For this review, take the finished solid that the model builds, in its own axes (mm). Face numbers are marked on the shaded views. A direction names the side the tool comes from. Give positions to 0.01 mm unless a question says otherwise; leave off trailing zeros. Loops run counter-clockwise (first coordinate to the right, second up) from the corner with the lowest first, then second, coordinate; pieces in that order, holes last. Notation, with made-up numbers: (-35.5, 66.25) -> (13.5, 66.25) arc R23 ccw to (13.5, 101.25) -> close; hole circle Ø11 at (12, 40.5). An arc over 180 degrees is marked (long way). Answer as CSV lines item,"result". Start each with the question number.
Item 1: For L1, parallel to Z at x = 0, y = -6; L2, parallel to Z at x = 1.75, y = 4; L3, parallel to X at y = 0.5, z = -1, list the stretches that pass through material, from the lowest coordinate up. Write a range as from..to.
Item 2: Clearance check with flat-ended pins moving along their axes: P1, Ø3, axis at y = -10, z = -6, coming from the +X side; P2, Ø3, axis at x = -2, y = -0.5, coming from the -Z side; P3, Ø8, axis at x = 2, y = -5, coming from the -Z side. State where each tip first meets the part, or that it passes through.
Item 3: Add section C-C on y = -5. State the section outline as (x, z) points.
Item 4: Add section B-B on z = 0. State the section outline as (x, y) points, plus the area to 3 significant figures.
Item 5: The part is to be moulded in two halves that separate along X. For the marked faces 3, 4 and 5, say which applies: +X half, -X half, draft (parallel to the pull), parting line (faces both ways), or undercut.
Item 6: Machinability: for the marked faces 1 and 2, which of the approach directions +Z, -Z, +X, -X, +Y, -Y give a long, thin tool a straight path to every point of the face, cutting with its end or side? Answer none if there is none.
Item 7: Add section D-D on z = 5.25. State the section outline as (x, y) points.
Item 8: Add section A-A on x = 0. State the section outline as (y, z) points.
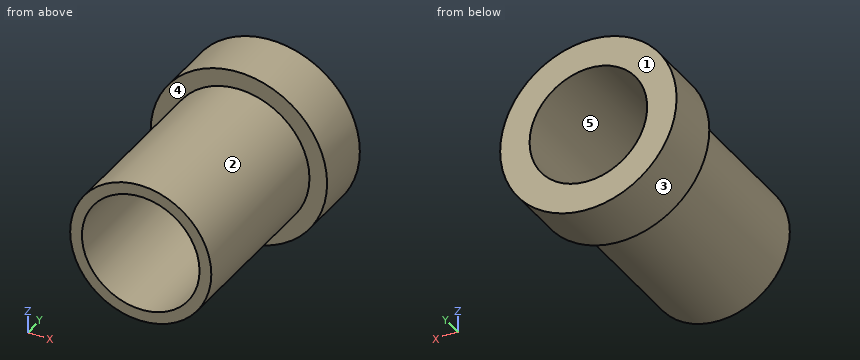
```python
from build123d import *

# Parameters (mm, degrees)
ESQUISSE1_R      = 7.5
EXTRUSION1_DEPTH = 5
ESQUISSE2_R      = 6
EXTRUSION2_DEPTH = 15
EXTRUSION3_REACH = 22
ESQUISSE3_R      = 5


with BuildPart() as part:
    # Esquisse1 → Extrusion1 (new body)
    with BuildSketch(Plane(origin=(0, 0, 0), x_dir=(1, 0, 0), z_dir=(0, 1, 0))):
        Circle(ESQUISSE1_R)
    extrude(amount=EXTRUSION1_DEPTH)

    # Esquisse2 → Extrusion2 (add)
    with BuildSketch(Plane.XZ):
        Circle(ESQUISSE2_R)
    extrude(amount=EXTRUSION2_DEPTH)

    # Esquisse3 → Extrusion3 (cut, up to next)
    with BuildSketch(Plane(origin=(0, 5, 0), x_dir=(1, 0, 0), z_dir=(0, 1, 0)), mode=Mode.PRIVATE) as extrusion3_sk1:
        Circle(ESQUISSE3_R)
    extrusion3_tool1 = extrude(extrusion3_sk1.sketch, amount=-EXTRUSION3_REACH, mode=Mode.PRIVATE) & part.part
    add(extrusion3_tool1.solids().sort_by_distance((0, 5, 0))[0], mode=Mode.SUBTRACT)


solid = part.part
```
Computed values:
1,L1,"-6..-5, 5..6"
1,L2,"-7.29..-4.68, 4.68..7.29"
1,L3,"-7.43..-4.9, 4.9..7.43"
2,P1,"x = 3.97"
2,P2,"z = -7.48"
2,P3,"z = -6"
3,outline,"circle Ø12 at (0, 0); hole circle Ø10 at (0, 0)"
4,outline,"(-7.5, 0) -> (-6, 0) -> (-6, -15) -> (-5, -15) -> (-5, 5) -> (-7.5, 5) -> close; (5, -15) -> (6, -15) -> (6, 0) -> (7.5, 0) -> (7.5, 5) -> (5, 5) -> close"
4,area,"55.0 mm²"
5,face 3,"parting line"
5,face 4,"draft"
5,face 5,"undercut"
6,face 1,"+Z, -Z, +X, -X, +Y"
6,face 2,"-Y"
7,outline,"(-5.36, 0) -> (-2.9, 0) -> (-2.9, -15) -> (2.9, -15) -> (2.9, 0) -> (5.36, 0) -> (5.36, 5) -> (-5.36, 5) -> close"
8,outline,"(-15, -6) -> (0, -6) -> (0, -7.5) -> (5, -7.5) -> (5, -5) -> (-15, -5) -> close; (-15, 5) -> (5, 5) -> (5, 7.5) -> (0, 7.5) -> (0, 6) -> (-15, 6) -> close"
